Study the drawing (mm; zero at the part's minimum x, y, z) and answer. A direction names the side the tool comes from. Round coordinates to 2 decimals unless told otherwise and drop trailing zeros. Write each loop counter-clockwise with the first axis right and the second up, starting at its lowest first coordinate (ties: lowest second). Pieces come first, ordered by that corner, then holes. Notation, with made-up numbers: (16.5, 37.5) -> (71.5, 37.5) arc R27 ccw to (71.5, 57.5) -> close; hole circle Ø7 at (37.25, -31). An arc over 180 degrees is marked (long way). Return JSON: item names as keys, results as strings.
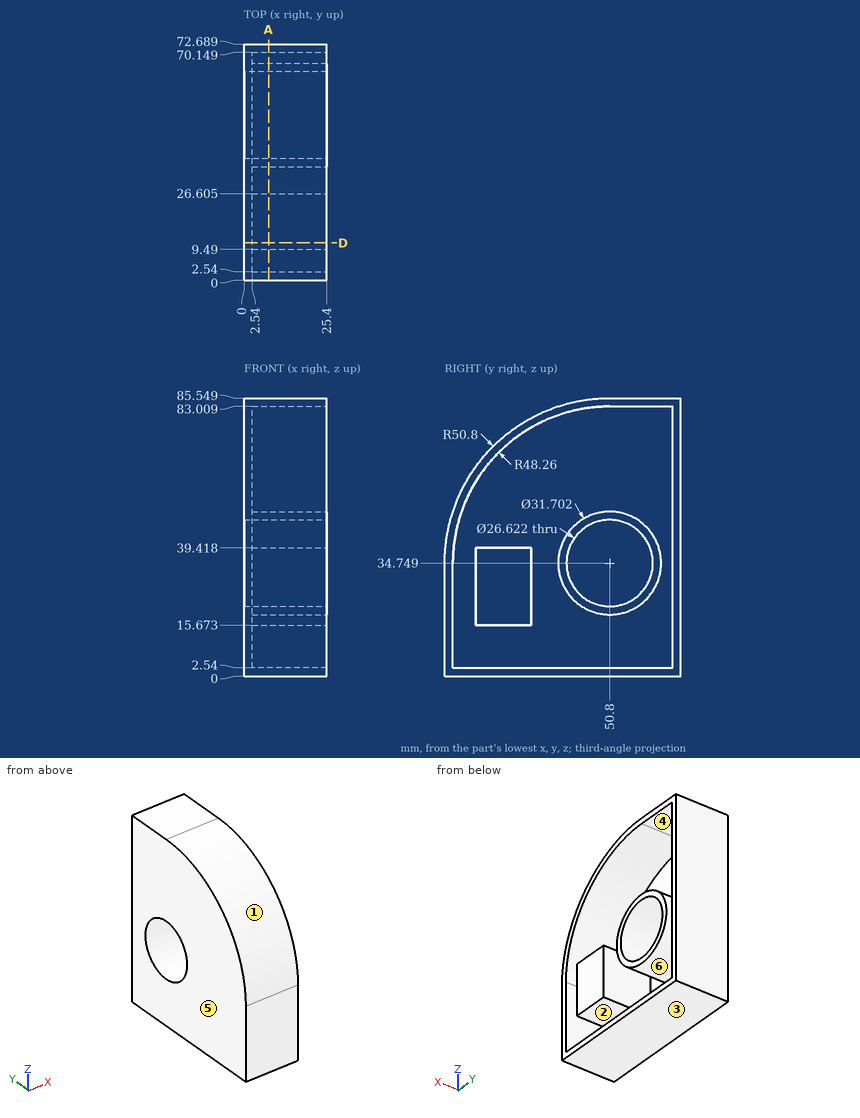
Item 1: A tool of negligible diameter and unlimited length cuts with its end or side. For the marked faces 5 and 6, from which of +Z, -Z, +X, -X, +Y, -Y can it reach the whole face along a straight path? Write none if from no direction.
Worked answers:
{"face 5": "+Z, -Z, -X, +Y, -Y", "face 6": "+X"}
Item 2: For a pull along Y with two mould halves and no side action, classify the marked faces 1, 2, 3 and 4 as released by +Y, released by -Y, zero draft, split by the parting line, or undercut.
Worked answers:
{"face 1": "released by -Y", "face 2": "undercut", "face 3": "zero draft", "face 4": "undercut"}
Item 3: Flat-ended cylindrical pins translate along their axes: pin 1 (1 mm diameter, centred on x = 21.5, y = 46, fed in from +Z); pin 2 (12 mm diameter, centred on x = 19.5, z = 58.5, fed in from -Y). Find the tip coordinate at first contact, or state that the pin passes through.
Worked answers:
{"pin 1": "stops at z = 85.37", "pin 2": "stops at y = 3.2"}
Item 4: Section A-A (x = 7.5) is taken. State how many separate pieces and enclosed holes the cut face has, then the cut area to 3 significant figures.
Worked answers:
{"separate pieces": "3", "enclosed holes": "2", "area": "1,360 mm2"}
Item 5: Straight lines are drawn through the part: L1, parallel to Z at x = 13.25, y = 50.8; L2, parallel to Z at x = 8.5, y = 70; L3, parallel to Y at x = 16.25, z = 6.5. For each, find the intervals that lie inside material, in ascending order. Write a range as [from, to].
Worked answers:
{"L1": "z = [0, 2.54], [18.9, 21.44], [48.06, 50.6], [83.01, 85.55]", "L2": "z = [0, 2.54], [83.01, 85.55]", "L3": "y = [0, 2.54], [70.15, 72.69]"}
Item 6: Section D-D (y = 11.5) is taken. Give the vertices of the cut face in (x, z).
Worked answers:
{"outline": "(0, 0) -> (25.4, 0) -> (25.4, 2.54) -> (2.54, 2.54) -> (2.54, 15.67) -> (25.4, 15.67) -> (25.4, 39.42) -> (2.54, 39.42) -> (2.54, 62.76) -> (25.4, 62.76) -> (25.4, 66.94) -> (0, 66.94) -> close"}
